from build123d import *

# Parameters (mm, degrees)
SKETCH1_R           = 36
BOSS_EXTRUDE1_DEPTH = 4
CUT_EXTRUDE1_DEPTH  = 52.068581339
SKETCH3_R           = 13.5
CUT_EXTRUDE2_DEPTH  = 52.068581339


with BuildPart() as part:
    # Sketch1 → Boss-Extrude1 (new body)
    with BuildSketch(Plane(origin=(0, 0, 0), x_dir=(1, 0, 0), z_dir=(0, 1, 0))):
        with Locations(Location((0, 0, 0), (0, 0, 270))):
            Circle(SKETCH1_R)
    extrude(amount=BOSS_EXTRUDE1_DEPTH)

    # Sketch2 → Cut-Extrude1 (cut, through all)
    with BuildSketch(Plane(origin=(0, 4, 0), x_dir=(1, 0, 0), z_dir=(0, 1, 0))):
        Polygon((-31.517749204, -2.278382028), (-27.535737886, -4.618663891), (-23.517988682, -2.340281863), (-23.482250796, 2.278382028), (-27.464262114, 4.618663891), (-31.482011318, 2.340281863), align=None)
        Polygon((27.5, -4.618802154), (31.5, -2.309401077), (31.5, 2.309401077), (27.5, 4.618802154), (23.5, 2.309401077), (23.5, -2.309401077), align=None)
    extrude(amount=-CUT_EXTRUDE1_DEPTH, mode=Mode.SUBTRACT)

    # Sketch3 → Cut-Extrude2 (cut, through all)
    with BuildSketch(Plane(origin=(0, 4, 0), x_dir=(1, 0, 0), z_dir=(0, 1, 0))):
        with Locations(Location((0, 0, 0), (0, 0, 270))):
            Circle(SKETCH3_R)
    extrude(amount=-CUT_EXTRUDE2_DEPTH, mode=Mode.SUBTRACT)


solid = part.part
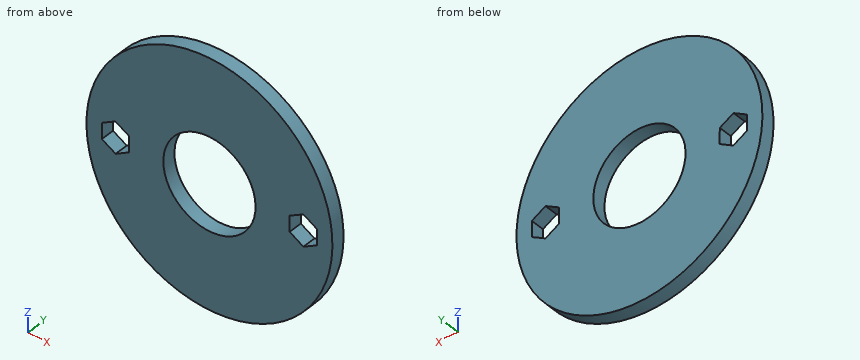
Geometry: final body of the model. Coordinates: model frame, mm. Give positions to 0.01 mm unless a question says otherwise; leave off trailing zeros. Write each loop counter-clockwise with the first axis right and the second up, starting at its lowest first coordinate (ties: lowest second). Pieces come first, ordered by that corner, then holes.
(1) Cut plane A-A, the plane y = 0.8. Return loops of the section in (x, z).
(2) First-contact query: P1, Ø8, axis at x = 8.5, z = -27.5, coming from the -Y side; P2, Ø2, axis at y = 1, z = -1, coming from the -X side. Flat tips, straight axial feed; report the tip coordinate or a pass-through.
(3) Ray query, line 1 (X direction, y = 2.1, z = 0); line 2 (X direction, y = 2.35, z = 2); line 3 (Z direction, x = -1.5, y = 3.45). Return the intervals inside material, ascending.
(4) Cut plane D-D, the plane x = -18. Return loops of the section in (y, z), then the cut area to 3 significant figures.
(5) Cut plane C-C, the plane z = -6. Return loops of the section in (x, y).
(6) Cut plane B-B, the plane x = 0. Return loops of the section in (y, z), then the cut area to 3 significant figures.
Values follow:
1. outline: circle Ø72 at (0, 0); hole (-31.52, 2.28) - (-31.48, -2.34) - (-27.46, -4.62) - (-23.48, -2.28) - (-23.52, 2.34) - (-27.54, 4.62) - close; hole circle Ø27 at (0, 0); hole (23.5, -2.31) - (27.5, -4.62) - (31.5, -2.31) - (31.5, 2.31) - (27.5, 4.62) - (23.5, 2.31) - close
2. P1: stops at y = 0
2. P2: stops at x = -36
3. line 1: x = -36 to -31.5, -23.5 to -13.5, 13.5 to 23.5, 31.5 to 36
3. line 2: x = -35.94 to -31.52, -23.52 to -13.35, 13.35 to 23.5, 31.5 to 35.94
3. line 3: z = -35.97 to -13.42, 13.42 to 35.97
4. outline: (0, -31.18) - (4, -31.18) - (4, 31.18) - (0, 31.18) - close
4. area: 249 mm2
5. outline: (-35.5, 0) - (-12.09, 0) - (-12.09, 4) - (-35.5, 4) - close; (12.09, 0) - (35.5, 0) - (35.5, 4) - (12.09, 4) - close
6. outline: (0, -36) - (4, -36) - (4, -13.5) - (0, -13.5) - close; (0, 13.5) - (4, 13.5) - (4, 36) - (0, 36) - close
6. area: 180 mm2
